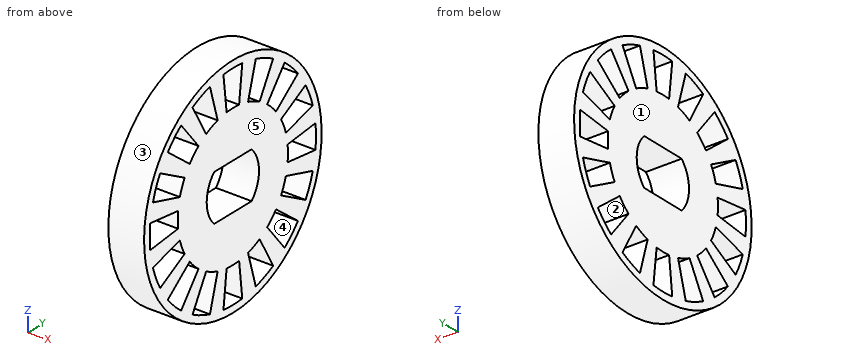
from build123d import *

# Parameters (mm, degrees)
SKETCH1_R           = 9.5
SKETCH1_R_2         = 2.8
BOSS_EXTRUDE1_DEPTH = 3
CUT_EXTRUDE2_DEPTH  = 3
CIRPATTERN1_COUNT   = 16


with BuildPart() as part:
    # Sketch1 → Boss-Extrude1 (new body)
    # profile 1 of 3: a face of its own
    with BuildSketch(Plane(origin=(0, 0, 0), x_dir=(0, 0, -1), z_dir=(1, 0, 0))):
        Circle(SKETCH1_R)
        Circle(SKETCH1_R_2, mode=Mode.SUBTRACT)
    # profile 2 of 3: a face of its own
    with BuildSketch(Plane(origin=(0, 0, 0), x_dir=(0, 0, -1), z_dir=(1, 0, 0))):
        with BuildLine():
            Line((1.95, 2.00935313), (1.95, -2.00935313))
            ThreePointArc((1.95, -2.00935313), (2.578759392, -1.090871211), (2.8, 0))
            ThreePointArc((2.8, 0), (2.578759392, 1.090871211), (1.95, 2.00935313))
        make_face()
    # profile 3 of 3: a face of its own
    with BuildSketch(Plane(origin=(0, 0, 0), x_dir=(0, 0, -1), z_dir=(1, 0, 0))):
        with BuildLine():
            ThreePointArc((-1.95, 2.00935313), (-2.8, 0), (-1.95, -2.00935313))
            Line((-1.95, -2.00935313), (-1.95, 2.00935313))
        make_face()
    extrude(amount=BOSS_EXTRUDE1_DEPTH)

    # Sketch3 → Cut-Extrude2 (cut)
    with BuildSketch(Plane(origin=(3, 0, 0), x_dir=(0, 0, -1), z_dir=(1, 0, 0))):
        with BuildLine():
            Line((-1.007508603, 8.842789516), (-0.667898961, 5.862073948))
            ThreePointArc((-0.667898961, 5.862073948), (0, 5.9), (0.667898961, 5.862073948))
            Line((0.667898961, 5.862073948), (1.007508603, 8.842789516))
            ThreePointArc((1.007508603, 8.842789516), (0, 8.9), (-1.007508603, 8.842789516))
        make_face()
    cut_extrude2 = extrude(amount=-CUT_EXTRUDE2_DEPTH, mode=Mode.SUBTRACT)

    # CirPattern1: Cut-Extrude2 ×16 about axis
    cirpattern1_axis = Axis((0, 0, 0), (1, 0, 0))
    for i in range(1, CIRPATTERN1_COUNT):
        add(cut_extrude2.rotate(cirpattern1_axis, i * 360 / CIRPATTERN1_COUNT), mode=Mode.SUBTRACT)


solid = part.part
The listing builds one solid part. Answer for the finished solid, in the listing's coordinates (mm). Face numbers are marked on the shaded views. A direction names the side the tool comes from. Round coordinates to 2 decimals unless told otherwise and drop trailing zeros. Write each loop counter-clockwise with the first axis right and the second up, starting at its lowest first coordinate (ties: lowest second). Pieces come first, ordered by that corner, then holes. Notation, with made-up numbers: M 53,83 L 93,83 A13 ccw 93,97 Z; hole C 43,87 d4. An arc over 180 degrees is marked long. Write each question's results on one line, items separated by ' | '. Start each with the question number.
(1) The part is cut by section A-A, the plane z = 0. Write down the section's boundary in (x, y), and give its area (3 significant figures).
(2) This flat-tipped pin is pushed along its axis until it touches: P1, Ø1.5, axis at x = 2, z = 3.5, coming from the -Y side. Where does it stop, or does it pass through?
(3) Find the intervals of material crossed by line 1 (Z direction, x = 2.25, y = -3); line 2 (Y direction, x = 0.95, z = -4.5); line 3 (Z direction, x = 1.95, y = -3.25), in increasing order.
(4) Determine the mould class of the marked faces 1, 2 and 3 for opening direction Y: +Y half, -Y half, draft (parallel to the pull), parting line (faces both ways), or undercut.
(5) The part is cut by section B-B, the plane y = 0. Write down the section's boundary in (x, z).
(6) For the marked faces 4 and 5, determine the directions among +Z, -Z, +X, -X, +Y, -Y from which every point of the face is accessible in a straight line to the end or side of a thin tool.
(7) The part is cut by section C-C, the plane x = 0.95. Give the number of separate pieces and of enclosed holes in the cut face, and give its area (3 significant figures).
Worked answers:
1) outline: M 0,-9.5 L 3,-9.5 L 3,-8.9 L 0,-8.9 Z; M 0,-5.9 L 3,-5.9 L 3,-2.8 L 0,-2.8 Z; M 0,2.8 L 3,2.8 L 3,5.9 L 0,5.9 Z; M 0,8.9 L 3,8.9 L 3,9.5 L 0,9.5 Z | area: 22.2 mm²
2) P1: stops at y = -9.09
3) line 1: z = -9.01 to -8.38, -5.41 to 5.41, 8.38 to 9.01 | line 2: y = -8.37 to -5.66, -3.82 to 3.82, 5.66 to 8.37 | line 3: z = -8.93 to -8.29, -5.86 to 5.86, 8.29 to 8.93
4) face 1: draft | face 2: undercut | face 3: parting line
5) outline: M 0,-9.5 L 3,-9.5 L 3,-8.9 L 0,-8.9 Z; M 0,-5.9 L 3,-5.9 L 3,-1.95 L 0,-1.95 Z; M 0,1.95 L 3,1.95 L 3,5.9 L 0,5.9 Z; M 0,8.9 L 3,8.9 L 3,9.5 L 0,9.5 Z
6) face 4: +X, -X | face 5: +Z, -Z, +X, +Y, -Y
7) separate pieces: 1 | enclosed holes: 17 | area: 183 mm²
